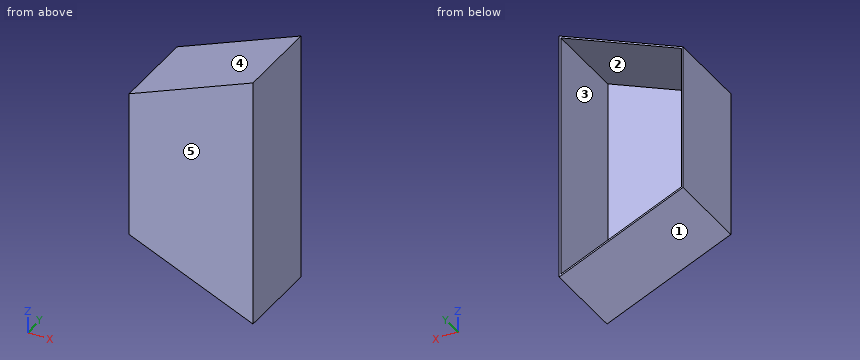
Autodesk Inventor part; units mm, degrees
ref_plane "YZ Plane" through (0, 0, 0) normal (1, 0, 0) x (0, 1, 0)
ref_plane "XZ Plane" through (0, 0, 0) normal (0, 1, 0) x (-1, 0, 0)
ref_plane "XY Plane" through (0, 0, 0) normal (0, 0, 1) x (1, 0, 0)
sketch "Sketch1" plane through (0, 0, 0) normal (0, 1, 0) x (-1, 0, 0)
  line L0 (0, 0) -> (0, -152.4)
  line L1 (0, -152.4) -> (74.791, -120.6531)
  line L2 (74.791, -120.6531) -> (74.791, -31.7531)
  line L3 (74.791, -31.7531) -> (0, 0)
  dimension "d5" = 152.4
  dimension "d6" = 81.25
  dimension "d7" = 67
  dimension "d8" = 88.9
extrude "Extrusion1" add sketch "Sketch1" along normal blind 50.8
shell "Shell1" thickness 1 removed faces 1 at (-24.9303, 50.8, -61.3844)
properties part number "footprint"
Could you check a few things on this model? Use its own coordinates, in mm. Face numbers are marked on the shaded views. A direction names the side the tool comes from. Coordinates: 2 decimals unless noted, no trailing zeros. Loops run counter-clockwise (first coordinate to the right, second up) from the corner with the lowest first, then second, coordinate; pieces in that order, holes last.
1. Imagine slicing it at C-C (x = -18.5). Please give me the cut outline in (y, z), and give its area (3 significant figures).
2. I need wall thicknesses on L1, parallel to X at y = 37, z = -67; L2, parallel to Y at x = -49.5, z = -37.5; L3, parallel to X at y = 20.5, z = -10. Which ranges of each line are inside material? Lowest first, please.
3. We'd pull the mould along X, two halves only. Please class the marked faces 3, 4 and 5: released by +X, released by -X, zero draft, split by the parting line, or undercut.
4. For the marked faces 1 and 2, which set-ups out of +Z, -Z, +X, -X, +Y, -Y let a thin tool reach every point of the face, with its end or its side?
5. Imagine slicing it at B-B (z = -86). Please give me the cut outline in (x, y), and give its area (3 significant figures).
6. Imagine slicing it at A-A (y = 23.5). Please give me the cut outline in (x, z).
7. For P1, Ø4, axis at x = -57.5, y = 7, coming from the +Z side; P2, Ø1, axis at x = -39, z = -41, coming from the +Y side; P3, Ø1, axis at x = -13.5, y = 25, coming from the -Z side, each with a flat end and sliding along its axis, tell me the tip position at first contact or that it passes through.
Computed values:
1. outline: (0, -144.55) - (50.8, -144.55) - (50.8, -143.46) - (1, -143.46) - (1, -8.94) - (50.8, -8.94) - (50.8, -7.85) - (0, -7.85) - close
1. area: 245 mm2
2. L1: x = -74.79 to -73.79, -1 to 0
2. L2: y = 0 to 1
2. L3: x = -23.55 to -21, -1 to 0
3. face 3: undercut
3. face 4: released by -X
3. face 5: zero draft
4. face 1: -Z, -X, +Y, -Y
4. face 2: +Y
5. outline: (-74.79, 0) - (0, 0) - (0, 50.8) - (-1, 50.8) - (-1, 1) - (-73.79, 1) - (-73.79, 50.8) - (-74.79, 50.8) - close
5. area: 174 mm2
6. outline: (-74.79, -120.65) - (0, -152.4) - (0, 0) - (-74.79, -31.75) - close; hole (-73.79, -119.99) - (-1, -150.89) - (-1, -1.51) - (-73.79, -32.41) - close
7. P1: stops at z = -23.56
7. P2: stops at y = 1
7. P3: stops at z = -146.88
